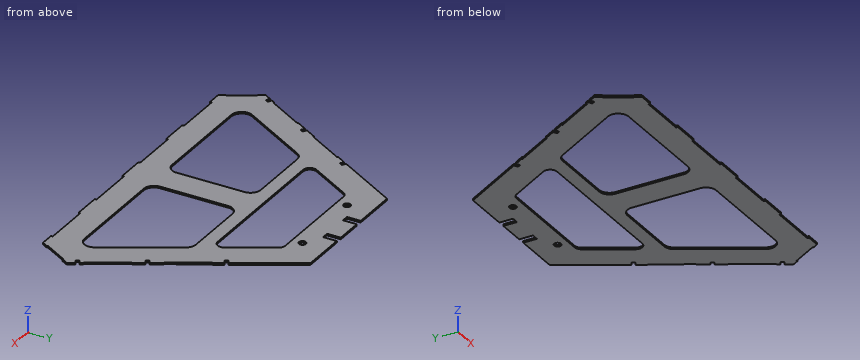
```python
from build123d import *

# Parameters (mm, degrees)
BOSS_EXTRUDE1_DEPTH = 3.175
SKETCH8_W           = 12.7
SKETCH8_H           = 25.4
CUT_EXTRUDE1_DEPTH  = 515.13014894
SKETCH9_W           = 88.9
SKETCH9_H           = 3.175
CUT_EXTRUDE2_DEPTH  = 515.13014894
CUT_EXTRUDE3_DEPTH  = 515.13014894
CUT_EXTRUDE4_DEPTH  = 515.13014894
CUT_EXTRUDE5_DEPTH  = 515.13014894
CUT_EXTRUDE6_DEPTH  = 515.13014894
CUT_EXTRUDE7_DEPTH  = 515.13014894
SKETCH15_R          = 6.35
CUT_EXTRUDE8_DEPTH  = 515.13014894


with BuildPart() as part:
    # Sketch7 → Boss-Extrude1 (new body)
    with BuildSketch(Plane.XY):
        Polygon((279.4, 0), (-279.4, 0), (-317.5, 65.991135768), (-122.138026348, 404.368), (122.138026348, 404.368), (317.5, 65.991135768), align=None)
    extrude(amount=BOSS_EXTRUDE1_DEPTH)

    # Sketch8 → Cut-Extrude1 (cut, through all)
    with BuildSketch(Plane.XY.offset(3.175)):
        with Locations((-31.75, 391.668)):
            Rectangle(SKETCH8_W, SKETCH8_H)
        with Locations((31.75, 391.668)):
            Rectangle(SKETCH8_W, SKETCH8_H)
    extrude(amount=-CUT_EXTRUDE1_DEPTH, mode=Mode.SUBTRACT)

    # Sketch9 → Cut-Extrude2 (cut, through all)
    with BuildSketch(Plane.XY.offset(3.175)):
        with Locations((-209.55, 1.5875)):
            Rectangle(SKETCH9_W, SKETCH9_H)
        with Locations((-69.85, 1.5875)):
            Rectangle(SKETCH9_W, SKETCH9_H)
        with Locations((69.85, 1.5875)):
            Rectangle(SKETCH9_W, SKETCH9_H)
        with Locations((209.55, 1.5875)):
            Rectangle(SKETCH9_W, SKETCH9_H)
    extrude(amount=-CUT_EXTRUDE2_DEPTH, mode=Mode.SUBTRACT)

    # Sketch10 → Cut-Extrude3 (cut, through all)
    with BuildSketch(Plane.XY.offset(3.175)):
        Polygon((-311.15, 54.99261314), (-309.775184671, 55.78636314), (-284.375184671, 11.792272628), (-285.75, 10.998522628), align=None)
        Polygon((285.75, 10.998522628), (311.15, 54.99261314), (309.775184671, 55.78636314), (284.375184671, 11.792272628), align=None)
    extrude(amount=-CUT_EXTRUDE3_DEPTH, mode=Mode.SUBTRACT)

    # Sketch11 → Cut-Extrude4 (cut, through all)
    with BuildSketch(Plane.XY.offset(3.175)):
        Polygon((-304.038, 89.30800374), (-302.663184671, 88.51425374), (-263.674184671, 156.045182676), (-265.049, 156.838932676), align=None)
        Polygon((-238.274184671, 200.039273188), (-199.285184671, 267.570202125), (-200.66, 268.363952125), (-239.649, 200.833023188), align=None)
        Polygon((304.038, 89.30800374), (302.663184671, 88.51425374), (263.674184671, 156.045182676), (265.049, 156.838932676), align=None)
        Polygon((239.649, 200.833023188), (238.274184671, 200.039273188), (199.285184671, 267.570202125), (200.66, 268.363952125), align=None)
    extrude(amount=-CUT_EXTRUDE4_DEPTH, mode=Mode.SUBTRACT)

    # Sketch12 → Cut-Extrude5 (cut, through all)
    with BuildSketch(Plane.XY.offset(3.175)):
        Polygon((-254.254, 175.536421144), (-247.379923357, 171.567671144), (-244.204923357, 177.066932458), (-251.079, 181.035682458), align=None)
        Polygon((251.079, 181.035682458), (254.254, 175.536421144), (247.379923357, 171.567671144), (244.204923357, 177.066932458), align=None)
        Polygon((-310.515, 78.089510659), (-303.640923357, 74.120760659), (-300.465923357, 79.620021973), (-307.34, 83.588771973), align=None)
        Polygon((-191.135, 284.861736067), (-184.260923357, 280.892986067), (-181.085923357, 286.392247381), (-187.96, 290.360997381), align=None)
        Polygon((307.34, 83.588771973), (310.515, 78.089510659), (303.640923357, 74.120760659), (300.465923357, 79.620021973), align=None)
        Polygon((187.96, 290.360997381), (191.135, 284.861736067), (184.260923357, 280.892986067), (181.085923357, 286.392247381), align=None)
    extrude(amount=-CUT_EXTRUDE5_DEPTH, mode=Mode.SUBTRACT)

    # Sketch13 → Cut-Extrude6 (cut, through all)
    with BuildSketch(Plane.XY.offset(3.175)):
        with BuildLine():
            Line((-92.808632673, 340.868), (92.808632673, 340.868))
            ThreePointArc((92.808632673, 340.868), (99.158632673, 339.166522628), (103.807155302, 334.518))
            Line((103.807155302, 334.518), (147.068010972, 259.588))
            ThreePointArc((147.068010972, 259.588), (147.068010972, 246.888), (136.069488344, 240.538))
            Line((136.069488344, 240.538), (-136.069488344, 240.538))
            ThreePointArc((-136.069488344, 240.538), (-147.068010972, 246.888), (-147.068010972, 259.588))
            Line((-147.068010972, 259.588), (-103.807155302, 334.518))
            ThreePointArc((-103.807155302, 334.518), (-99.158632673, 339.166522628), (-92.808632673, 340.868))
        make_face()
    extrude(amount=-CUT_EXTRUDE6_DEPTH, mode=Mode.SUBTRACT)

    # Sketch14 → Cut-Extrude7 (cut, through all)
    with BuildSketch(Plane.XY.offset(3.175)):
        with BuildLine():
            Line((45.361818975, 215.138), (161.732707809, 215.138))
            ThreePointArc((161.732707809, 215.138), (171.257707809, 212.585783942), (178.230491751, 205.613))
            Line((178.230491751, 205.613), (251.114035033, 79.375))
            ThreePointArc((251.114035033, 79.375), (251.114035033, 60.325), (234.616251091, 50.8))
            Line((234.616251091, 50.8), (45.361818975, 50.8))
            ThreePointArc((45.361818975, 50.8), (31.891434794, 56.379615818), (26.311818975, 69.85))
            Line((26.311818975, 69.85), (26.311818975, 196.088))
            ThreePointArc((26.311818975, 196.088), (31.891434794, 209.558384182), (45.361818975, 215.138))
        make_face()
        with BuildLine():
            Line((-161.732707809, 215.138), (-45.361818975, 215.138))
            ThreePointArc((-45.361818975, 215.138), (-31.891434794, 209.558384182), (-26.311818975, 196.088))
            Line((-26.311818975, 196.088), (-26.311818975, 69.85))
            ThreePointArc((-26.311818975, 69.85), (-31.891434794, 56.379615818), (-45.361818975, 50.8))
            Line((-45.361818975, 50.8), (-234.616251091, 50.8))
            ThreePointArc((-234.616251091, 50.8), (-251.114035033, 60.325), (-251.114035033, 79.375))
            Line((-251.114035033, 79.375), (-178.230491751, 205.613))
            ThreePointArc((-178.230491751, 205.613), (-171.257707809, 212.585783942), (-161.732707809, 215.138))
        make_face()
    extrude(amount=-CUT_EXTRUDE7_DEPTH, mode=Mode.SUBTRACT)

    # Sketch15 → Cut-Extrude8 (cut, through all)
    with BuildSketch(Plane(origin=(0, 0, 0), x_dir=(-1, 0, 0), z_dir=(0, 0, -1))):
        with Locations((-71.338026348, 359.918)):
            Circle(SKETCH15_R)
        with Locations(Location((71.338026348, 359.918, 0), (0, 0, 180))):
            Circle(SKETCH15_R)
    extrude(amount=-CUT_EXTRUDE8_DEPTH, mode=Mode.SUBTRACT)


solid = part.part
```
Geometry check sheet. Reference: the model listing, model coordinates, mm. Coordinates: 2 decimals unless noted, no trailing zeros. Order: outer loops, then holes, each group sorted by start corner. A loop starts at its lowest first (then second) coordinate and runs counter-clockwise, first axis right, second up.
Q1. Sectioned sample at C-C on y = 327. Record the cut outline in (x, z) (3 decimals), and give its area (3 significant figures).
Reply:
outline: (-166.806, 0) - (-108.148, 0) - (-108.148, 3.175) - (-166.806, 3.175) - close; (108.148, 0) - (166.806, 0) - (166.806, 3.175) - (108.148, 3.175) - close
area: 372 mm2
Q2. Depth check by flat-ended pin: pin 1 Ø1 at (y, z) = (1, 1.5) entering from +X; pin 2 Ø1 at (x, z) = (104.5, 1.5) entering from -Y (3 decimals); pin 3 Ø7.5 at (x, y) = (71.34, 359.92) entering from -Z; pin 4 Ø1.6 at (y, z) = (148, 1.5) entering from -X. Enter the tip coordinate at first touch or a pass-through.
Reply:
pin 1: stops at x = 280.27
pin 2: stops at y = 3.175
pin 3: passes through
pin 4: stops at x = -268.78
Q3. Thickness scan on probe 1 along Y at (x, z) = (21, 1.2); probe 2 along Y at (x, z) = (162.5, 2.1); probe 3 along X at (y, z) = (107.5, 0.3). Record the ranges inside material, lowest first.
Reply:
probe 1: y = 0 to 240.54, 340.87 to 404.37
probe 2: y = 0 to 50.8, 215.12 to 334.46
probe 3: x = -291.7 to -234.88, -26.31 to 26.31, 234.88 to 291.7
Q4. Sectioned sample at A-A on x = 17. Record the cut outline in (y, z) (3 decimals), and give its area (3 significant figures).
Reply:
outline: (0, 0) - (240.538, 0) - (240.538, 3.175) - (0, 3.175) - close; (340.868, 0) - (404.368, 0) - (404.368, 3.175) - (340.868, 3.175) - close
area: 965 mm2
Q5. Sectioned sample at B-B on y = 98. Record the cut outline in (x, z) (3 decimals), and give its area (3 significant figures).
Reply:
outline: (-297.187, 0) - (-240.361, 0) - (-240.361, 3.175) - (-297.187, 3.175) - close; (-26.312, 0) - (26.312, 0) - (26.312, 3.175) - (-26.312, 3.175) - close; (240.361, 0) - (297.187, 0) - (297.187, 3.175) - (240.361, 3.175) - close
area: 528 mm2
Q6. Sectioned sample at D-D on z = 2.6. Give the number of separate pieces and of enclosed holes in the cut face, and give its area (3 significant figures).
Reply:
separate pieces: 1
enclosed holes: 5
area: 96,600 mm2
